Model file for the job. Use its own axes, mm. Face numbers are marked on the shaded views. Round coordinates to 2 decimals unless told otherwise and drop trailing zeros. Order: outer loops, then holes, each group sorted by start corner. A loop starts at its lowest first (then second) coordinate and runs counter-clockwise, first axis right, second up. Notation, with made-up numbers: (42.25, -20) - (90.25, -20) arc R5 cw to (90.25, -15) - close; hole circle Ø6 at (14, -24.5). An arc over 180 degrees is marked (long way). Write item = value, one per line.
```python
from build123d import *

# Parameters (mm, degrees)
EXTRUDE_1_DEPTH     = 6
CUT_EXTRUDE_1_DEPTH = 3.8
CUT_EXTRUDE_2_DEPTH = 49.87803699
SKETCH_3_W          = 18.536502565
SKETCH_3_H          = 15.637579157
CUT_EXTRUDE_3_DEPTH = 4
SKETCH_4_W          = 6
SKETCH_4_H          = 10
EXTRUDE_2_DEPTH     = 19.25
SKETCH_5_R          = 0.85
CUT_EXTRUDE_4_DEPTH = 50.639324129
SKETCH_7_W          = 12.8
SKETCH_7_H          = 11.8
EXTRUDE_3_DEPTH     = 1.9
SKETCH_8_W          = 12
SKETCH_8_H          = 10
CUT_EXTRUDE_5_DEPTH = 5
CUT_EXTRUDE_6_DEPTH = 5
CHAMFER_1_SIZE      = 0.5
SKETCH_10_W         = 1.9
SKETCH_10_H         = 2
EXTRUDE_4_DEPTH     = 5.9
CHAMFER_2_SIZE      = 6
CUT_EXTRUDE_7_DEPTH = 2.1
CUT_EXTRUDE_START   = -10
CUT_EXTRUDE_8_DEPTH = 2.1
CHAMFER_3_SIZE      = 0.6


with BuildPart() as part:
    # 草图1 → 凸台-拉伸1 (new body)
    with BuildSketch(Plane(origin=(0, 0, 0), x_dir=(0, 0, -1), z_dir=(1, 0, 0))):
        Polygon((-25, 5), (25, 5), (25, 3), (48.25, 3), (48.25, -3), (25, -3), (25, -5), (-25, -5), (-25, -3), (-48.25, -3), (-48.25, 3), (-25, 3), align=None)
    extrude(amount=-EXTRUDE_1_DEPTH)

    # 草图1<3> → 切除-拉伸1 (cut)
    with BuildSketch(Plane(origin=(0, 0, 0), x_dir=(0, 0, -1), z_dir=(1, 0, 0))):
        with BuildLine():
            Line((-15.5, 2.25), (15.5, 2.25))
            ThreePointArc((15.5, 2.25), (17.75, 0), (15.5, -2.25))
            Line((15.5, -2.25), (-15.5, -2.25))
            ThreePointArc((-15.5, -2.25), (-17.75, 0), (-15.5, 2.25))
        make_face()
    extrude(amount=-CUT_EXTRUDE_1_DEPTH, mode=Mode.SUBTRACT)

    # 草图1<4> → 切除-拉伸2 (cut, through all)
    with BuildSketch(Plane(origin=(0, 0, 0), x_dir=(0, 0, -1), z_dir=(1, 0, 0))):
        with BuildLine():
            Line((-12.3, 2.25), (12.3, 2.25))
            ThreePointArc((12.3, 2.25), (14.55, 0), (12.3, -2.25))
            Line((12.3, -2.25), (-12.3, -2.25))
            ThreePointArc((-12.3, -2.25), (-14.55, 0), (-12.3, 2.25))
        make_face()
    extrude(amount=-CUT_EXTRUDE_2_DEPTH, mode=Mode.SUBTRACT)

    # 草图3 → 切除-拉伸3 (cut)
    with BuildSketch(Plane(origin=(0, 0, -48.25), x_dir=(-1, 0, 0), z_dir=(0, 0, -1))):
        with Locations((1.626975839, 1.766046581)):
            Rectangle(SKETCH_3_W, SKETCH_3_H)
    extrude(amount=-CUT_EXTRUDE_3_DEPTH, mode=Mode.SUBTRACT)

    # 草图4 → 凸台-拉伸2 (add)
    with BuildSketch(Plane(origin=(0, 0, -25), x_dir=(-1, 0, 0), z_dir=(0, 0, -1))):
        with Locations((3, 0)):
            Rectangle(SKETCH_4_W, SKETCH_4_H)
    extrude(amount=EXTRUDE_2_DEPTH)

    # 草图5 → 切除-拉伸4 (cut, through all)
    with BuildSketch(Plane.XZ.offset(5)):
        with Locations(Location((-2.8, 29.1, 0), (0, 0, 270))):
            Circle(SKETCH_5_R)
        with Locations(Location((-2.8, -19.9, 0), (0, 0, 270))):
            Circle(SKETCH_5_R)
    extrude(amount=-CUT_EXTRUDE_4_DEPTH, mode=Mode.SUBTRACT)

    # 草图7 → 凸台-拉伸3 (add)
    with BuildSketch(Plane(origin=(0, 0, -44.25), x_dir=(-1, 0, 0), z_dir=(0, 0, -1))):
        with Locations((-0.4, 0)):
            Rectangle(SKETCH_7_W, SKETCH_7_H)
    extrude(amount=EXTRUDE_3_DEPTH)

    # 草图8 → 切除-拉伸5 (cut)
    with BuildSketch(Plane(origin=(0, 0, 0), x_dir=(0, 0, -1), z_dir=(1, 0, 0))):
        with Locations((38.25, 0)):
            Rectangle(SKETCH_8_W, SKETCH_8_H)
    extrude(amount=-CUT_EXTRUDE_5_DEPTH, mode=Mode.SUBTRACT)

    # 草图9 → 切除-拉伸6 (cut)
    with BuildSketch(Plane.XY.offset(-44.25)):
        with BuildLine():
            Line((12.6, -3.55), (1, -3.55))
            ThreePointArc((1, -3.55), (-2.55, 0), (1, 3.55))
            Line((1, 3.55), (12.6, 3.55))
            ThreePointArc((12.6, 3.55), (16.15, 0), (12.6, -3.55))
        make_face()
    extrude(amount=-CUT_EXTRUDE_6_DEPTH, mode=Mode.SUBTRACT)

    # 倒角1
    chamfer_1_edges = [part.edges().sort_by_distance(p)[0] for p in [
        (3.9, 3.55, -44.25),
        (3.9, -3.55, -44.25),
        (-2.55, 0, -44.25),
    ]]
    chamfer(chamfer_1_edges, length=CHAMFER_1_SIZE)

    # 草图10 → 凸台-拉伸4 (add)
    with BuildSketch(Plane.ZY.offset(6)):
        with Locations((-45.2, 6.9)):
            Rectangle(SKETCH_10_W, SKETCH_10_H)
        with Locations((-45.2, -6.9)):
            Rectangle(SKETCH_10_W, SKETCH_10_H)
    extrude(amount=-EXTRUDE_4_DEPTH)

    # 倒角2
    chamfer_2_edges = [part.edges().sort_by_distance(p)[0] for p in [
        (0, 4, 25),
        (0, -4, 25),
    ]]
    chamfer(chamfer_2_edges, length=CHAMFER_2_SIZE - 0.0001)  # a hair under: the kernel refuses the full size

    # 草图11 → 切除-拉伸7 (cut)
    with BuildSketch(Plane(origin=(0, 5, 0), x_dir=(1, 0, 0), z_dir=(0, 1, 0))):
        Polygon((0, 24.514101615), (-6, 21.05), (-6, 17.55), (0, 17.55), align=None)
    extrude(amount=-CUT_EXTRUDE_7_DEPTH, mode=Mode.SUBTRACT)

    # 草图11<2> → 切除-拉伸8 (cut)
    with BuildSketch(Plane(origin=(0, 5, 0), x_dir=(1, 0, 0), z_dir=(0, 1, 0)).offset(CUT_EXTRUDE_START)):
        Polygon((0, 24.514101615), (-6, 21.05), (-6, 17.55), (0, 17.55), align=None)
    extrude(amount=CUT_EXTRUDE_8_DEPTH, mode=Mode.SUBTRACT)

    # 倒角3
    chamfer_3_edges = [part.edges().sort_by_distance(p)[0] for p in [
        (0, 3, 33.62505),
        (0, -3, 33.62505),
        (0, 2.9, -21.032050808),
        (0, -2.9, -21.032050808),
    ]]
    chamfer(chamfer_3_edges, length=CHAMFER_3_SIZE)


solid = part.part
```
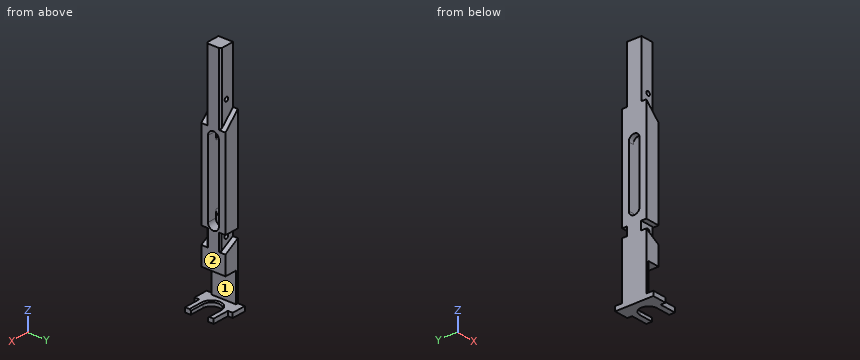
1) Cut at A-A (y = 0). Write the cut outline in (x, z).
Conclusion:
outline = (-6, -46.15) - (-2.55, -46.15) - (-2.55, -44.75) - (-3.05, -44.25) - (-5, -44.25) - (-5, -32.25) - (0, -32.25) - (0, -17.75) - (-3.8, -17.75) - (-3.8, -14.55) - (-6, -14.55) - close; (-6, 14.55) - (-3.8, 14.55) - (-3.8, 17.75) - (0, 17.75) - (0, 48.25) - (-6, 48.25) - close; hole circle Ø1.7 at (-2.8, -19.9); hole circle Ø1.7 at (-2.8, 29.1)
2) Flat gauge pins, fed straight in: pin 1 Ø6 at (x, z) = (-3.5, -22) entering from -Y; pin 2 Ø6.5 at (x, z) = (-3, -1.5) entering from +Y; pin 3 Ø1 at (y, z) = (0, -14) entering from +X (3 decimals); pin 4 Ø1 at (x, z) = (5, -45.5) entering from -Y. Where does each tip first touch, or does it go through?
Conclusion:
pin_1 = -5
pin_2 = 5
pin_3 = through
pin_4 = -5.9
3) Cut at D-D (z = 21). Write the cut outline in (x, y), and give its area (3 significant figures).
Conclusion:
outline = (-6, -5) - (-2, -5) - (-2, -3) - (-0.6, -3) - (0, -2.4) - (0, 2.4) - (-0.6, 3) - (-2, 3) - (-2, 5) - (-6, 5) - close
area = 51.6 mm^2
4) Cut at C-C (z = -19.9). Write the cut outline in (x, y).
Conclusion:
outline = (-6, -2.9) - (-3.65, -2.9) - (-3.65, 2.9) - (-6, 2.9) - close; (-1.95, -2.9) - (-0.6, -2.9) - (0, -2.3) - (0, 2.3) - (-0.6, 2.9) - (-1.95, 2.9) - close
5) Wall check: line 1 along Y through (x, z) = (-1.5, -7); line 2 along X through (y, z) = (-0.8, 29.1); line 3 along Z through (x, y) = (-2.5, 1). Give the ranges that are in metal, low to high.
Conclusion:
line_1 = -5 to -2.25, 2.25 to 5
line_2 = -6 to -3.65, -1.95 to 0
line_3 = -46.15 to -44.66, -32.25 to -20.7, -19.1 to -17.52, 17.52 to 28.3, 29.9 to 48.25
6) Cut at B-B (x = 5.5). Write the cut outline in (y, z).
Conclusion:
outline = (-5.9, -46.15) - (-3.55, -46.15) - (-3.55, -44.75) - (-4.05, -44.25) - (-5.9, -44.25) - close; (3.55, -46.15) - (5.9, -46.15) - (5.9, -44.25) - (4.05, -44.25) - (3.55, -44.75) - close
7) Mould opens along Z. For the marked faces 1 and 2 say: +Z half, -Z half, draft (parallel to the pull), parting line (faces both ways), or undercut.
Conclusion:
face_1 = undercut
face_2 = draft
